```python
from build123d import *

# Parameters (mm, degrees)
SKETCH1_R           = 7.5
SKETCH1_R_2         = 2.5
BOSS_EXTRUDE1_DEPTH = 130
SKETCH2_R           = 2
CUT_EXTRUDE1_DEPTH  = 16


with BuildPart() as part:
    # Sketch1 → Boss-Extrude1 (new body)
    with BuildSketch(Plane.XY):
        Circle(SKETCH1_R)
        Circle(SKETCH1_R_2, mode=Mode.SUBTRACT)
    extrude(amount=BOSS_EXTRUDE1_DEPTH)

    # Sketch2 → Cut-Extrude1 (cut)
    with BuildSketch(Plane.ZY.offset(7.5)):
        with Locations((20, 0)):
            Circle(SKETCH2_R)
        with Locations((40, 0)):
            Circle(SKETCH2_R)
    extrude(amount=-CUT_EXTRUDE1_DEPTH, mode=Mode.SUBTRACT)


solid = part.part
```
CAD build for the part. Positions are in the model's coordinates, mm. Give positions to 0.01 mm unless a question says otherwise; leave off trailing zeros. Loops run counter-clockwise (first coordinate to the right, second up) from the corner with the lowest first, then second, coordinate; pieces in that order, holes last. Notation, with made-up numbers: (30, 17) - (51, 17) arc R35 ccw to (51, 52) - close; hole circle Ø8 at (32, 61). An arc over 180 degrees is marked (long way). Put each result on its own line as item: value.
Q1. Slice it at A-A (y = 0). Give the cut face in (x, z).
Filled in:
outline: (-7.5, 0) - (-2.5, 0) - (-2.5, 18) - (-7.5, 18) - close; (-7.5, 22) - (-2.5, 22) - (-2.5, 38) - (-7.5, 38) - close; (-7.5, 42) - (-2.5, 42) - (-2.5, 130) - (-7.5, 130) - close; (2.5, 0) - (7.5, 0) - (7.5, 18) - (2.5, 18) - close; (2.5, 22) - (7.5, 22) - (7.5, 38) - (2.5, 38) - close; (2.5, 42) - (7.5, 42) - (7.5, 130) - (2.5, 130) - close
Q2. Slice it at B-B (x = 0). Give the cut face in (y, z).
Filled in:
outline: (-7.5, 0) - (-2.5, 0) - (-2.5, 130) - (-7.5, 130) - close; (2.5, 0) - (7.5, 0) - (7.5, 130) - (2.5, 130) - close
Q3. Probe line 1 along Z through (x, y) = (4, 0); line 2 along Y through (x, z) = (0, 62). List the from-to ranges inside material, lowest first.
Filled in:
line 1: z = 0 to 18, 22 to 38, 42 to 130
line 2: y = -7.5 to -2.5, 2.5 to 7.5
Q4. Slice it at C-C (z = 20). Give the cut face in (x, y).
Filled in:
outline: (-7.23, -2) arc R7.5 ccw to (7.23, -2) - (1.5, -2) arc R2.5 cw to (-1.5, -2) - close; (-7.23, 2) - (-1.5, 2) arc R2.5 cw to (1.5, 2) - (7.23, 2) arc R7.5 ccw to start
Q5. Flat gauge pins, fed straight in: pin 1 (1.5 mm diameter, centred on y = 4.5, z = 63, fed in from +X); pin 2 (1 mm diameter, centred on y = 3, z = 28, fed in from -X); pin 3 (2 mm diameter, centred on y = 5, z = 34, fed in from +X). Where does each tip first touch, or does it go through?
Filled in:
pin 1: stops at x = 6.5
pin 2: stops at x = -7.07
pin 3: stops at x = 6.34
Q6. Mould opens along Y. For faces 1 (the face through (-4.543, -0.766, 41.847)), 2 (the face through (6.93, -2.87, 64.09)), 3 (the face through (-2, 2, 0)) say: pulls with the +Y half, pulls with the -Y half, needs draft (parallel to the pull), parting line crosses it, or undercut.
Filled in:
face 1: undercut
face 2: parting line crosses it
face 3: needs draft
Q7. Slice it at D-D (x = 6.25). Give the cut face in (y, z), plus the area to 3 significant figures.
Filled in:
outline: (-4.15, 0) - (4.15, 0) - (4.15, 130) - (-4.15, 130) - close; hole circle Ø4 at (0, 20); hole circle Ø4 at (0, 40)
area: 1,050 mm²
